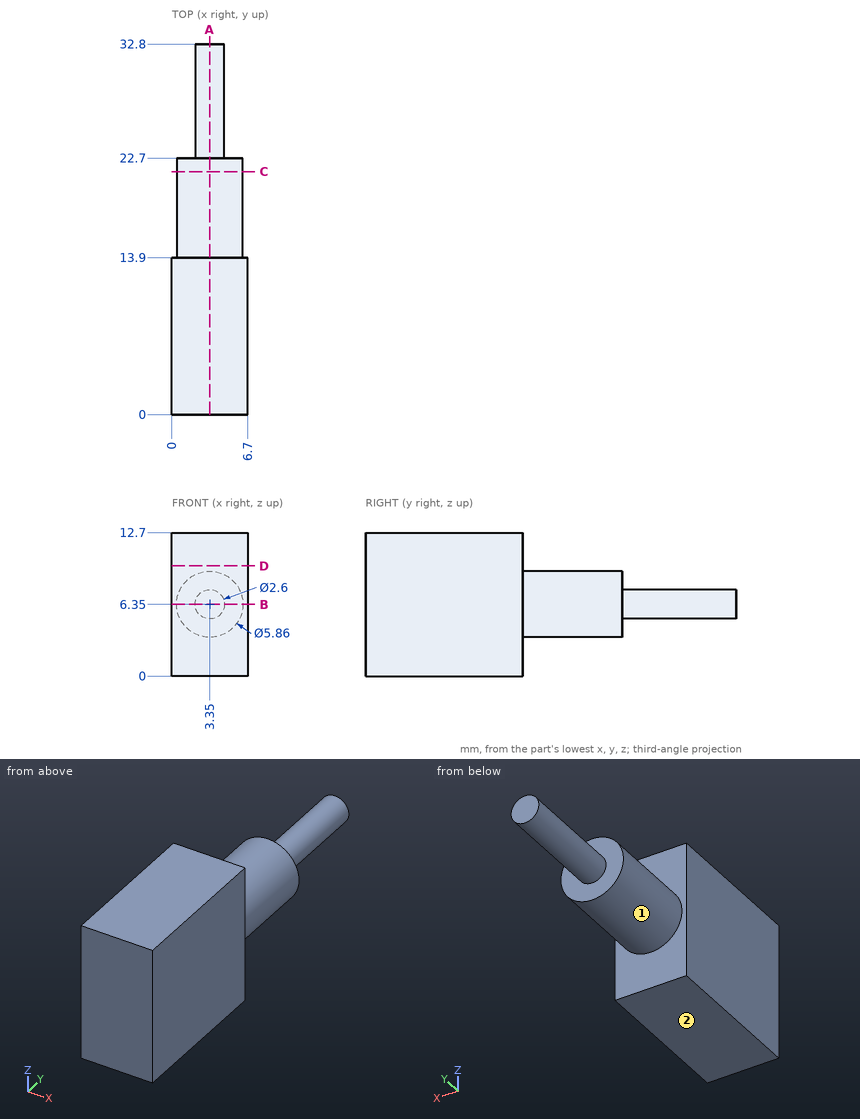
Design review of the part shown in the three views and the two pictorial views. Dimensions are in mm from the part's minimum x, y and z. A direction names the side the tool comes from. Give positions to 0.01 mm unless a question says otherwise; leave off trailing zeros. Write each loop counter-clockwise with the first axis right and the second up, starting at its lowest first coordinate (ties: lowest second). Pieces come first, ordered by that corner, then holes. Notation, with made-up numbers: (-21.75, 14) - (29.25, 14) arc R12 ccw to (29.25, 24) - close; hole circle Ø3 at (0.25, 37.25). An arc over 180 degrees is marked (long way). Return JSON: item names as keys, results as strings. Group by question number.
(1) We need section C-C, the plane y = 21.5. Give the boundary of the cut face in (x, z).
(2) We need section B-B, the plane z = 6.35. Give the boundary of the cut face in (x, y), then the cut area to 3 significant figures.
(3) Machinability: for the marked faces 1 and 2, which of the approach directions +Z, -Z, +X, -X, +Y, -Y give a long, thin tool a straight path to every point of the face, cutting with its end or side? Answer none if there is none.
(4) Insertion check: pin 1 (2 mm diameter, centred on x = 6, z = 5, fed in from +Y); pin 2 (3 mm diameter, centred on x = 3.5, y = 22, fed in from +Z); pin 3 (3 mm diameter, centred on y = 28.5, z = 4, fed in from -X). Each pin has a flat end and moves straight along its axis. Give the tip position at first contact, or say it passes through.
(5) We need section D-D, the plane z = 9.75. Give the boundary of the cut face in (x, y), then the cut area to 3 significant figures.
(6) To check wall thickness, follow probe 1 along Y at (x, z) = (1.5, 1.25); probe 2 along Y at (x, z) = (4.75, 5.5); probe 3 along Z at (x, y) = (1.25, 22.5). State the ranges of each line that lie inside material, in increasing order.
(7) We need section A-A, the plane x = 3.35. Give the boundary of the cut face in (y, z), then the cut area to 3 significant figures.
Reported:
{
 "1": {"outline": "circle Ø5.86 at (3.35, 6.35)"},
 "2": {"outline": "(0, 0) - (6.7, 0) - (6.7, 13.9) - (6.28, 13.9) - (6.28, 22.7) - (4.65, 22.7) - (4.65, 32.8) - (2.05, 32.8) - (2.05, 22.7) - (0.42, 22.7) - (0.42, 13.9) - (0, 13.9) - close", "area": "171 mm2"},
 "3": {"face 1": "+Y", "face 2": "-Z, +X, -X, +Y, -Y"},
 "4": {"pin 1": "stops at y = 22.7", "pin 2": "stops at z = 9.28", "pin 3": "stops at x = 2.37"},
 "5": {"outline": "(0, 0) - (6.7, 0) - (6.7, 13.9) - (0, 13.9) - close", "area": "93.1 mm2"},
 "6": {"probe 1": "y = 0 to 13.9", "probe 2": "y = 0 to 22.7", "probe 3": "z = 4.31 to 8.39"},
 "7": {"outline": "(0, 0) - (13.9, 0) - (13.9, 3.42) - (22.7, 3.42) - (22.7, 5.05) - (32.8, 5.05) - (32.8, 7.65) - (22.7, 7.65) - (22.7, 9.28) - (13.9, 9.28) - (13.9, 12.7) - (0, 12.7) - close", "area": "254 mm2"}
}
